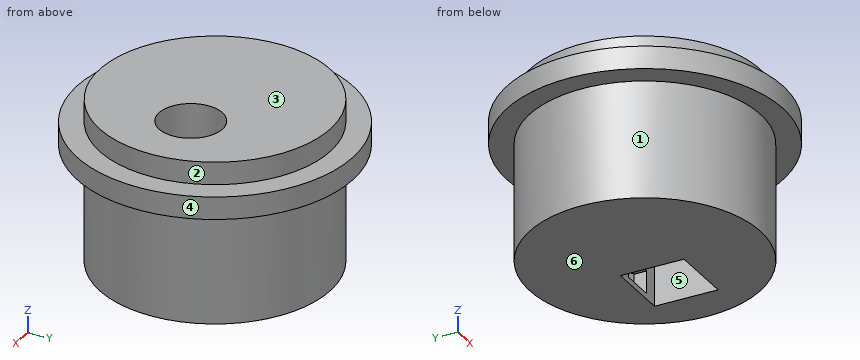
```python
from build123d import *

# Parameters (mm, degrees)
SKETCH5_W           = 42.1
SKETCH5_H           = 42.1
SKETCH5_W_2         = 28.1
SKETCH5_H_2         = 28.1
BOSS_EXTRUDE3_DEPTH = 32
CUT_EXTRUDE2_REACH  = 80.495
SKETCH6_W           = 15
SKETCH6_H           = 10
SKETCH7_W           = 42.1
SKETCH7_H           = 42.1
SKETCH7_R           = 14.05
BOSS_EXTRUDE4_DEPTH = 40
CUT_EXTRUDE3_START  = -72
CUT_EXTRUDE3_DEPTH  = 72
CIRPATTERN1_COUNT   = 4
BOSS_EXTRUDE6_START = -72
SKETCH24_R          = 51.05
SKETCH24_R_2        = 21.05
BOSS_EXTRUDE6_DEPTH = 72
BOSS_EXTRUDE7_START = -20
SKETCH25_R          = 61.05
SKETCH25_R_2        = 51.05
BOSS_EXTRUDE7_DEPTH = 10


with BuildPart() as part:
    # Sketch5 → Boss-Extrude3 (new body)
    with BuildSketch(Plane.XY.offset(20)):
        with Locations((20, 0)):
            Rectangle(SKETCH5_W, SKETCH5_H)
        with Locations((20, 0)):
            Rectangle(SKETCH5_W_2, SKETCH5_H_2, mode=Mode.SUBTRACT)
    extrude(amount=BOSS_EXTRUDE3_DEPTH)

    # Sketch6 → Cut-Extrude2 (cut, up to next)
    with BuildSketch(Plane(origin=(0, 21.05, 0), x_dir=(1, 0, 0), z_dir=(0, 1, 0)), mode=Mode.PRIVATE) as cut_extrude2_sk1:
        with Locations((20, -27.5)):
            Rectangle(SKETCH6_W, SKETCH6_H)
    cut_extrude2_tool1 = extrude(cut_extrude2_sk1.sketch, amount=-CUT_EXTRUDE2_REACH, mode=Mode.PRIVATE) & part.part
    add(cut_extrude2_tool1.solids().sort_by_distance((20, 21.05, 27.5))[0], mode=Mode.SUBTRACT)

    # Sketch7 → Boss-Extrude4 (add)
    with BuildSketch(Plane.XY.offset(52)):
        with Locations((20, 0)):
            Rectangle(SKETCH7_W, SKETCH7_H)
        with Locations((20, 0)):
            Circle(SKETCH7_R, mode=Mode.SUBTRACT)
    extrude(amount=BOSS_EXTRUDE4_DEPTH)

    # Sketch11 → Cut-Extrude3 (cut)
    with BuildSketch(Plane.XY.offset(92).offset(CUT_EXTRUDE3_START)):
        with BuildLine():
            Line((20, 21.05), (-1.05, 21.05))
            Line((-1.05, 21.05), (-1.05, 0))
            ThreePointArc((-1.05, 0), (5.115402256, 14.884597744), (20, 21.05))
        make_face()
    cut_extrude3 = extrude(amount=CUT_EXTRUDE3_DEPTH, mode=Mode.SUBTRACT)

    # CirPattern1: Cut-Extrude3 ×4 about axis
    cirpattern1_axis = Axis((20, 0, 92), (0, 0, 1))
    for i in range(1, CIRPATTERN1_COUNT):
        add(cut_extrude3.rotate(cirpattern1_axis, i * 360 / CIRPATTERN1_COUNT), mode=Mode.SUBTRACT)

    # Sketch24 → Boss-Extrude6 (add)
    with BuildSketch(Plane.XY.offset(92).offset(BOSS_EXTRUDE6_START)):
        Circle(SKETCH24_R)
        with Locations((20, 0)):
            Circle(SKETCH24_R_2, mode=Mode.SUBTRACT)
    extrude(amount=BOSS_EXTRUDE6_DEPTH)

    # Sketch25 → Boss-Extrude7 (add)
    with BuildSketch(Plane.XY.offset(92).offset(BOSS_EXTRUDE7_START)):
        Circle(SKETCH25_R)
        Circle(SKETCH25_R_2, mode=Mode.SUBTRACT)
    extrude(amount=BOSS_EXTRUDE7_DEPTH)


solid = part.part
```
CAD build for the part. Positions are in the model's coordinates, mm. Face numbers are marked on the shaded views. A direction names the side the tool comes from. Coordinates: 2 decimals unless noted, no trailing zeros. Order: outer loops, then holes, each group sorted by start corner. A loop starts at its lowest first (then second) coordinate and runs counter-clockwise, first axis right, second up. Notation, with made-up numbers: (20, 3.25) - (51, 3.25) arc R18 ccw to (51, 14.25) - close; hole circle Ø4 at (53.5, -35.5). An arc over 180 degrees is marked (long way). Answer in a Markdown table with one row per item.
1. Slice it at D-D, the plane z = 50.5. List the corners of the cut face in (x, y).
Answer:
| item | result |
|---|---|
| outline | circle Ø102.1 at (0, 0); hole (5.95, -14.05) - (34.05, -14.05) - (34.05, 14.05) - (5.95, 14.05) - close |
2. Slice it at B-B, the plane z = 29. List the corners of the cut face in (x, y), then the cut area to 3 significant figures.
Answer:
| item | result |
|---|---|
| outline | circle Ø102.1 at (0, 0); hole (5.95, -14.05) - (34.05, -14.05) - (34.05, 14.05) - (27.5, 14.05) - (27.5, 19.67) arc R21.05 ccw to (12.5, 19.67) - (12.5, 14.05) - (5.95, 14.05) - close |
| area | 7,300 mm² |
3. Pull direction Y, two halves, no side cores. Call the marked faces 4, 5 and 6: +Y half, -Y half, draft (parallel to the pull), parting line (faces both ways), or undercut.
Answer:
| item | result |
|---|---|
| face 4 | parting line |
| face 5 | undercut |
| face 6 | draft |
4. 3-axis set-ups, long thin cutter, end or side, ignore diameter. For the marked faces 1, 2 and 3: which of +Z, -Z, +X, -X, +Y, -Y reach the whole face in a straight line?
Answer:
| item | result |
|---|---|
| face 1 | -Z |
| face 2 | +Z |
| face 3 | +Z, +X, -X, +Y, -Y |
5. Flat gauge pins, fed straight in: P1, Ø8.5, axis at y = -1, z = 42, coming from the +X side; P2, Ø10, axis at y = 24, z = 44, coming from the -X side; P3, Ø6, axis at y = 18, z = 30, coming from the -X side. Where does each tip first touch, or does it go through?
Answer:
| item | result |
|---|---|
| P1 | x = 51.05 |
| P2 | x = -47.38 |
| P3 | x = -48.8 |
6. Slice it at A-A, the plane x = 0. List the corners of the cut face in (y, z), then the cut area to 3 significant figures.
Answer:
| item | result |
|---|---|
| outline | (-61.05, 72) - (-51.05, 72) - (-51.05, 20) - (51.05, 20) - (51.05, 72) - (61.05, 72) - (61.05, 82) - (51.05, 82) - (51.05, 92) - (-51.05, 92) - (-51.05, 82) - (-61.05, 82) - close |
| area | 7,550 mm² |
7. Slice it at C-C, the plane y = -4.5. List the corners of the cut face in (x, z), then the cut area to 3 significant figures.
Answer:
| item | result |
|---|---|
| outline | (-60.88, 72) - (-50.85, 72) - (-50.85, 20) - (5.95, 20) - (5.95, 52) - (6.69, 52) - (6.69, 92) - (-50.85, 92) - (-50.85, 82) - (-60.88, 82) - close; (33.31, 52) - (34.05, 52) - (34.05, 20) - (50.85, 20) - (50.85, 72) - (60.88, 72) - (60.88, 82) - (50.85, 82) - (50.85, 92) - (33.31, 92) - close |
| area | 5,560 mm² |
8. Drill centre lines: L1, parallel to Z at x = 28, y = -45; L2, parallel to Y at x = 20, z = 68; L3, parallel to X at y = -37.5, z = 79. Where is each one in solid material? Low to high. Write a range as from..to.
Answer:
| item | result |
|---|---|
| L1 | 72..82 |
| L2 | -46.97..-14.05, 14.05..46.97 |
| L3 | -48.18..48.18 |
